Input: dimensioned drawing with shaded views. Units: mm. Origin: part minimum x, y, z. Give positions to 0.01 mm unless a question says otherwise; leave off trailing zeros. Loops run counter-clockwise (first coordinate to the right, second up) from the corner with the lowest first, then second, coordinate; pieces in that order, holes last.
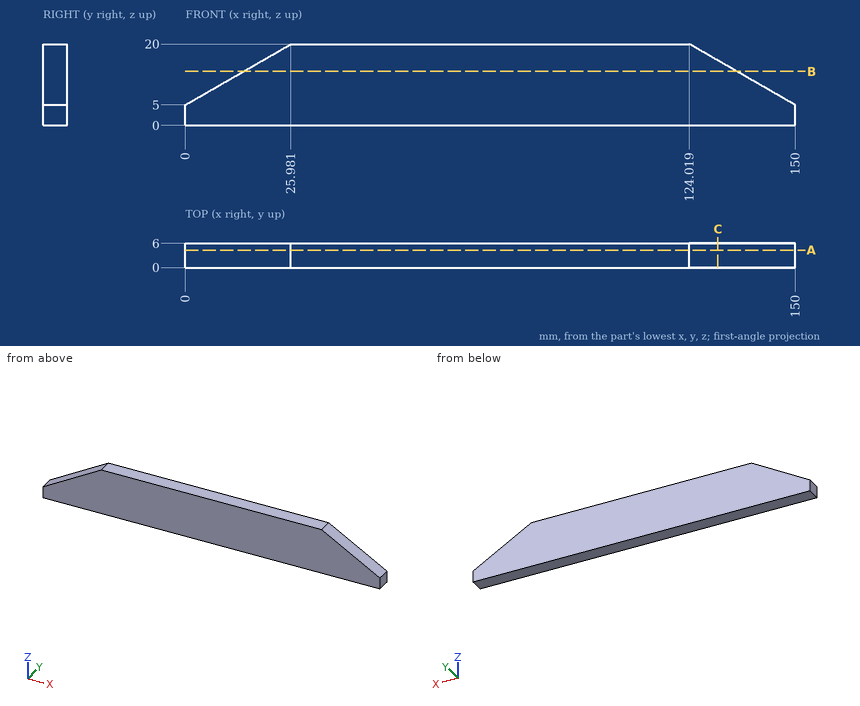
Item 1: Ray query, probe 1 along X at (y, z) = (1.65, 13.75) (1 decimal); probe 2 along X at (y, z) = (3.4, 18.75) (1 decimal); probe 3 along Z at (x, y) = (131, 3.1). Return the intervals inside material, ascending.
Values follow:
probe 1: x = 15.2 to 134.8
probe 2: x = 23.8 to 126.2
probe 3: z = 0 to 15.97
Item 2: Section query C-C on x = 131. Return loops of the section in (y, z).
Values follow:
outline: (0, 0) - (6, 0) - (6, 15.97) - (0, 15.97) - close
Item 3: Section query A-A on y = 4.3. Return loops of the section in (x, z).
Values follow:
outline: (0, 0) - (150, 0) - (150, 5) - (124.02, 20) - (25.98, 20) - (0, 5) - close
Item 4: Section query B-B on z = 13.25. Return loops of the section in (x, y).
Values follow:
outline: (14.29, 0) - (135.71, 0) - (135.71, 6) - (14.29, 6) - close
Item 5: Pin query (flat end, axial travel): pin 1 (1 mm diameter, centred on y = 1.5, z = 8, fed in from -X); pin 2 (1.5 mm diameter, centred on x = 128, y = 1, fed in from -Z); pin 3 (1 mm diameter, centred on y = 1.5, z = 8.5, fed in from -X) (1 decimal). Return the tip coordinate at first contact, or that it passes through.
Values follow:
pin 1: stops at x = 4.33
pin 2: stops at z = 0
pin 3: stops at x = 5.2
